from build123d import *

# Parameters (mm, degrees)
F0_R     = 25
F0_R_2   = 10
F1_DEPTH = 10
F3_DEPTH = 25
F4_COUNT = 40


with BuildPart() as f1:
    # F0 (on Front) → F1 (new body)
    with BuildSketch(Plane.XZ):
        Circle(F0_R)
        Circle(F0_R_2, mode=Mode.SUBTRACT)
    extrude(amount=F1_DEPTH)

    # F2 (on face) → F3 (cut)
    with BuildSketch(Plane.XZ.offset(10)):
        with BuildLine():
            Line((-0.5, 22.45), (0, 22.45))
            Line((0, 22.45), (0.5, 22.45))
            Line((0.5, 22.45), (1.4135669538, 24.9600045767))
            ThreePointArc((1.4135669538, 24.9600045767), (0, 25), (-1.4135669538, 24.9600045767))
            Line((-1.4135669538, 24.9600045767), (-0.5, 22.45))
        make_face()
    f3 = extrude(amount=-F3_DEPTH, mode=Mode.SUBTRACT)

    # F4: F3 ×40 about axis
    f4_axis = Axis((0, 0, 0), (0, 1, 0))
    for i in range(1, F4_COUNT):
        add(f3.rotate(f4_axis, i * 360 / F4_COUNT), mode=Mode.SUBTRACT)


solid = f1.part
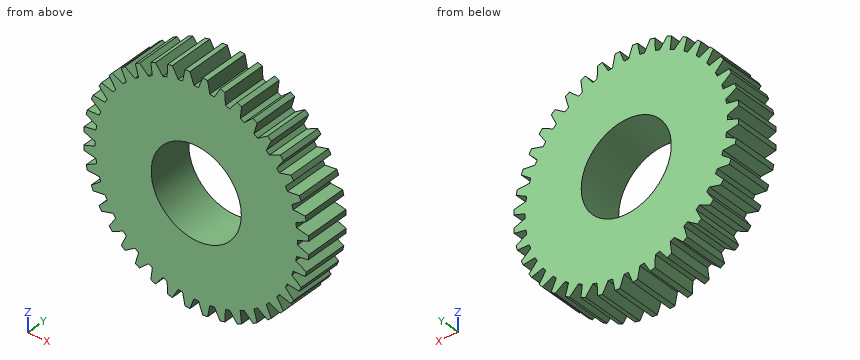
Source: CAD feature listing. Evaluate the final solid. Frame: model axes, mm. Round coordinates to 2 decimals unless told otherwise and drop trailing zeros. Loops run counter-clockwise (first coordinate to the right, second up) from the corner with the lowest first, then second, coordinate; pieces in that order, holes last. Notation, with made-up numbers: (10.25, 26) -> (31.25, 26) arc R29 cw to (31.25, 54) -> close; hole circle Ø3 at (67.5, 25.25). An arc over 180 degrees is marked (long way). Answer as a JSON object with one key per item and string values. Group by question number.
Q1. Section query B-B (z = 14.5). Output: boundary loops of the cut face in (x, y).
Q2. Section query A-A (x = 11.5). Output: boundary loops of the cut face in (y, z).
Q3. Ray query, line 1 (Z direction, x = -16.5, y = -4.25); line 2 (X direction, y = -7.25, z = 21); line 3 (X direction, y = -4.25, z = -19). Return the intervals inside material, ascending. Write a range as from..to.
Q4. Contact query for flat-ended pins moving along their axis: P1, Ø1, axis at x = 14.5, y = -3.5, coming from the -Z side; P2, Ø2, axis at y = -8.5, z = -5.5, coming from the +X side; P3, Ø12, axis at x = 0, z = 0, coming from the -Y side; P4, Ø1, axis at x = -2.5, z = 16.5, coming from the +Y side. Output: stop coordinate, or through.
Completed:
{
 "1": {"outline": "(-18.48, -10) -> (18.48, -10) -> (18.48, 0) -> (-18.48, 0) -> close"},
 "2": {"outline": "(-10, -20.58) -> (0, -20.58) -> (0, 20.58) -> (-10, 20.58) -> close"},
 "3": {"line 1": "-18.78..-18.33, -15.65..15.65, 18.33..18.78", "line 2": "-13.52..-11.95, -9.84..9.84, 11.95..13.52", "line 3": "-16.25..-15.28, -12.95..12.95, 15.28..16.25"},
 "4": {"P1": "z = -18.81", "P2": "x = 24.43", "P3": "through", "P4": "y = 0"}
}
